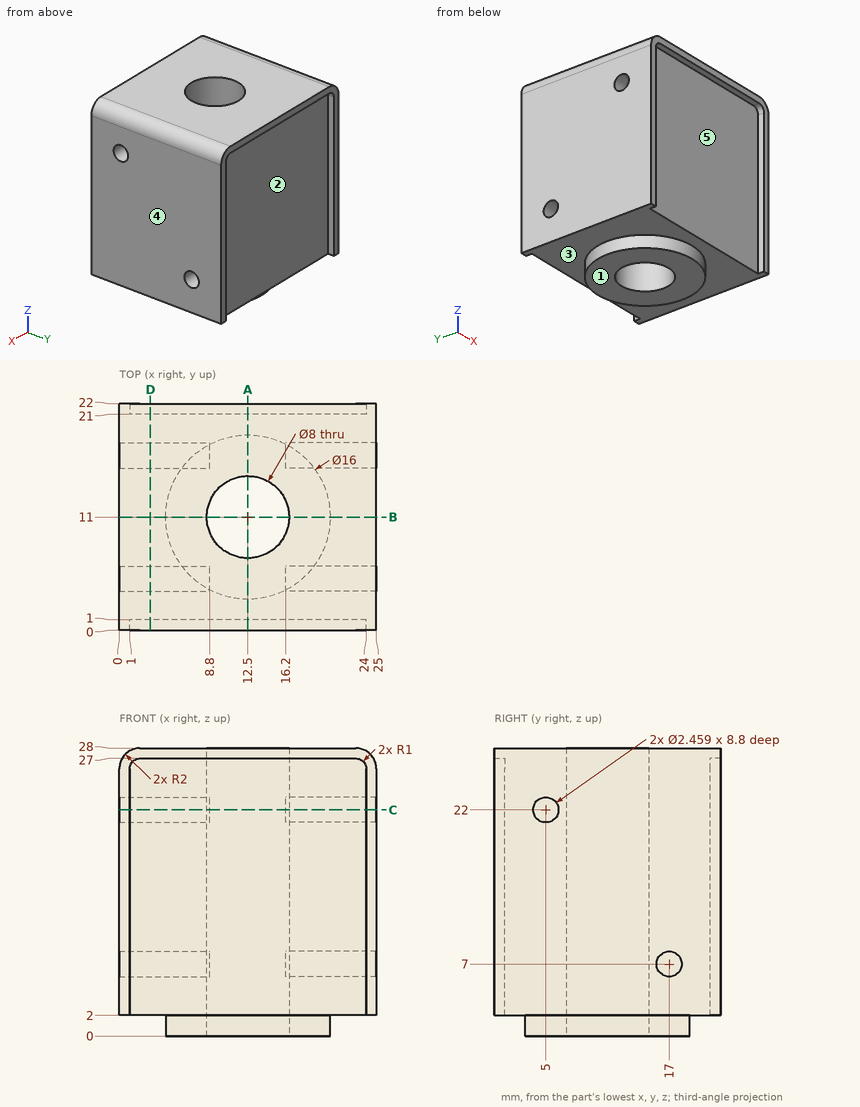
Source: three-view drawing plus pictorial views. Frame: mm from the lowest corner of the part. A direction names the side the tool comes from. Give positions to 0.01 mm unless a question says otherwise; leave off trailing zeros. Write each loop counter-clockwise with the first axis right and the second up, starting at its lowest first coordinate (ties: lowest second). Pieces come first, ordered by that corner, then holes.
(1) Access query for the marked faces 1 and 2. Directions: +Z, -Z, +X, -X, +Y, -Y. A direction counts if a zero-diameter tool reaches every point of the face in a straight line with its end or side. Return the directions, or none.
(2) Cut plane D-D, the plane x = 3. Return loops of the section in (y, z), then the cut area to 3 significant figures.
(3) Cut plane A-A, the plane x = 12.5. Return loops of the section in (y, z), then the cut area to 3 significant figures.
(4) Mould query, pull axis X, two halves, no side actions, for the marked faces 3, 4 and 5. Classes: released by +X, released by -X, zero draft, split by the parting line, or undercut.
(5) First-contact query: P1, Ø1.5, axis at x = 10.5, y = 6, coming from the -Z side; P2, Ø6, axis at x = 17.5, z = 16.5, coming from the -Y side; P3, Ø2, axis at y = 17, z = 7, coming from the -X side; P4, Ø1.1, axis at x = 12, y = 21.5, coming from the -Z side. Flat tips, straight axial feed; report the tip coordinate or a pass-through.
(6) Cut plane C-C, the plane z = 22. Return loops of the section in (x, y).
(7) Ray query, line 1 (Z direction, x = 23, y = 17); line 2 (Y direction, x = 3.75, z = 7); line 3 (Y direction, x = 6, z = 22). Return the intervals inside material, ascending.
(8) Cut plane B-B, the plane y = 11. Return loops of the section in (x, z), then the cut area to 3 significant figures.
Values follow:
1. face 1: -Z, +X, -X, +Y, -Y
1. face 2: -Z, +Y
2. outline: (0, 27) - (1, 27) - (1, 2) - (21, 2) - (21, 27) - (22, 27) - (22, 28) - (0, 28) - close; hole circle Ø2.46 at (5, 22); hole circle Ø2.46 at (17, 7)
2. area: 513 mm2
3. outline: (0, 27) - (1, 27) - (1, 2) - (3, 2) - (3, 0) - (7, 0) - (7, 28) - (0, 28) - close; (15, 0) - (19, 0) - (19, 2) - (21, 2) - (21, 27) - (22, 27) - (22, 28) - (15, 28) - close
3. area: 330 mm2
4. face 3: zero draft
4. face 4: released by +X
4. face 5: undercut
5. P1: stops at z = 0
5. P2: stops at y = 1
5. P3: stops at x = 8.8
5. P4: stops at z = 2
6. outline: (0, 0) - (1, 0) - (1, 1) - (24, 1) - (24, 0) - (25, 0) - (25, 3.77) - (16.2, 3.77) - (16.2, 6.23) - (25, 6.23) - (25, 22) - (24, 22) - (24, 21) - (1, 21) - (1, 22) - (0, 22) - (0, 6.23) - (8.8, 6.23) - (8.8, 3.77) - (0, 3.77) - close; hole circle Ø8 at (12.5, 11)
7. line 1: z = 2 to 5.77, 8.23 to 28
7. line 2: y = 1 to 15.77, 18.23 to 21
7. line 3: y = 1 to 3.77, 6.23 to 21
8. outline: (0, 2) - (4.5, 2) - (4.5, 0) - (8.5, 0) - (8.5, 28) - (2, 28) arc R2 ccw to (0, 26) - close; (16.5, 0) - (20.5, 0) - (20.5, 2) - (25, 2) - (25, 26) arc R2 ccw to (23, 28) - (16.5, 28) - close
8. area: 456 mm2
